Check sheet for the modelled part. Datum: model origin and axes. Units: mm. Round coordinates to 2 decimals unless told otherwise and drop trailing zeros. Write each loop counter-clockwise with the first axis right and the second up, starting at its lowest first coordinate (ties: lowest second). Pieces come first, ordered by that corner, then holes. Notation, with made-up numbers: M 85,11 L 127,11 A25 cw 127,33 Z; hole C -18.5,32.25 d2. An arc over 180 degrees is marked long. One line per item, written item: value.
Autodesk Inventor part; units mm, degrees
ref_plane "YZ Plane" through (0, 0, 0) normal (1, 0, 0) x (0, 1, 0)
ref_plane "XZ Plane" through (0, 0, 0) normal (0, 1, 0) x (-1, 0, 0)
ref_plane "XY Plane" through (0, 0, 0) normal (0, 0, 1) x (1, 0, 0)
sketch "Sketch1" plane through (0, 0, 0) normal (0, 0, 1) x (1, 0, 0)
  circle A0 centre (0, 5) radius 7.5
  line L0 (42.7333, 18.5) -> (-42.7333, 18.5)
  line L1 (-42.7333, -29) -> (42.7333, -29)
  circle A1 centre (18.5, 5) radius 2.25
  circle A2 centre (-18.5, 5) radius 2.25
  circle A3 centre (30.8333, 5) radius 3.9
  circle A4 centre (-30.8333, 5) radius 3.9
  line L2 (42.7333, 18.5) -> (42.7333, -29)
  line L3 (-42.7333, -29) -> (-42.7333, 18.5)
  circle A5 centre (0, 5) radius 13.5 construction
  line L4 (0, 41.7106) -> (0, -39.2634) construction
  dimension "d2" = 4.5
  dimension "d3" = 4.5
  dimension "d4" = 7.8
  dimension "d5" = 7.8
  dimension "d48" = 47.5
  dimension "d58" = 15
  dimension "d63" = 27
  dimension "d75" = 34
  dimension "d76" = 30.8333
  dimension "d77" = 85.4667
  dimension "d93" = 47.5
  dimension "d99" = 61.667
extrude "Extrusion1" add sketch "Sketch1" against normal blind 3
sketch "Sketch4" plane through (0, 0, 0) normal (0, 0, 1) x (1, 0, 0)
  line L0 (42.7333, 18.5) -> (39.7333, 18.5)
  line L1 (-42.7333, 18.5) -> (-39.7333, 18.5)
  line L2 (42.7333, -29) -> (21.3667, -29)
  line L3 (21.3667, -26) -> (39.7333, -26)
  line L4 (-42.7333, -29) -> (-21.3667, -29)
  line L5 (-21.3667, -29) -> (-21.3667, -26)
  line L6 (-21.3667, -26) -> (-39.7333, -26)
  line L7 (-42.7333, -23) -> (-42.7333, -29)
  line L8 (42.7333, 18.5) -> (39.7333, 18.5)
  line L9 (39.7333, 18.5) -> (39.7333, 2.6667)
  line L10 (39.7333, 2.6667) -> (42.7333, 2.6667)
  line L11 (42.7333, 2.6667) -> (42.7333, 18.5)
  line L12 (39.7333, -26) -> (39.7333, -13.1667)
  line L13 (39.7333, -13.1667) -> (42.7333, -13.1667)
  line L14 (-42.7333, 2.6667) -> (-39.7333, 2.6667)
  line L15 (-39.7333, 2.6667) -> (-39.7333, 18.5)
  line L16 (-39.7333, 18.5) -> (-42.7333, 18.5)
  line L17 (-42.7333, 18.5) -> (-42.7333, 2.6667)
  line L18 (-42.7333, -29) -> (-39.7333, -29)
  line L19 (-39.7333, -26) -> (-39.7333, -13.1667)
  line L20 (-39.7333, -13.1667) -> (-42.7333, -13.1667)
  line L21 (-42.7333, -13.1667) -> (-42.7333, -29)
  line L22 (21.3667, -29) -> (21.3667, -26)
  line L23 (-21.3667, -23) -> (-21.3667, -29)
  line L24 (-42.7333, 18.5) -> (-39.7333, 18.5)
  line L25 (-42.7333, -29) -> (42.7333, -29)
  line L26 (42.7333, 18.5) -> (-42.7333, 18.5)
  line L27 (50.1623, -5.25) -> (-50.4474, -5.25) construction
  line L28 (42.7333, -29) -> (42.7333, 18.5)
  line L29 (42.7333, -3.75) -> (34.7333, -3.75)
  line L30 (34.7333, -3.75) -> (34.7333, -6.75)
  line L31 (34.7333, -6.75) -> (42.7333, -6.75)
  line L32 (42.7333, -6.75) -> (42.7333, -3.75)
  circle A0 centre (0, 5) radius 13.5 construction
  circle A1 centre (0, 5) radius 7.5
  line L33 (42.7333, -2.6) -> (39.7333, -2.6)
  line L34 (39.7333, -2.6) -> (39.7333, -7.9)
  line L35 (39.7333, -7.9) -> (42.7333, -7.9)
  line L36 (42.7333, -7.9) -> (42.7333, -2.6)
  line L37 (35.3333, -2.6) -> (37.7333, -2.6)
  line L38 (37.7333, -2.6) -> (37.7333, -7.9)
  line L39 (37.7333, -7.9) -> (35.3333, -7.9)
  line L40 (35.3333, -7.9) -> (35.3333, -2.6)
  line L41 (0, 33.7344) -> (0, -36.9537) construction
  line L42 (-42.7333, 18.5) -> (-42.7333, -29)
  line L43 (-42.7333, -3.75) -> (-34.7333, -3.75)
  line L44 (-34.7333, -3.75) -> (-34.7333, -6.75)
  line L45 (-34.7333, -6.75) -> (-42.7333, -6.75)
  line L46 (-42.7333, -6.75) -> (-42.7333, -3.75)
  line L47 (-42.7333, -2.6) -> (-39.7333, -2.6)
  line L48 (-39.7333, -2.6) -> (-39.7333, -7.9)
  line L49 (-39.7333, -7.9) -> (-42.7333, -7.9)
  line L50 (-42.7333, -7.9) -> (-42.7333, -2.6)
  line L51 (-35.3333, -2.6) -> (-37.7333, -2.6)
  line L52 (-37.7333, -2.6) -> (-37.7333, -7.9)
  line L53 (-37.7333, -7.9) -> (-35.3333, -7.9)
  line L54 (-35.3333, -7.9) -> (-35.3333, -2.6)
  line L55 (42.7333, -29) -> (-42.7333, -29)
  line L56 (-1.5, -29) -> (1.5, -29)
  line L57 (1.5, -29) -> (1.5, -21)
  line L58 (1.5, -21) -> (-1.5, -21)
  line L59 (-1.5, -21) -> (-1.5, -29)
  line L60 (-2.65, -29) -> (2.65, -29)
  line L61 (2.65, -29) -> (2.65, -26)
  line L62 (2.65, -26) -> (-2.65, -26)
  line L63 (-2.65, -26) -> (-2.65, -29)
  line L64 (-2.65, -21.6) -> (2.65, -21.6)
  line L65 (2.65, -21.6) -> (2.65, -24)
  line L66 (2.65, -24) -> (-2.65, -24)
  line L67 (-2.65, -24) -> (-2.65, -21.6)
  line L68 (31.3, 16) -> (24.0167, 16) construction
  line L69 (11.4333, 16) -> (11.4333, 13) construction
  line L70 (11.4333, 13) -> (18.7167, 13) construction
  line L71 (31.3, 13) -> (31.3, 16) construction
  circle A2 centre (30.8333, 5) radius 3.9
  line L72 (21.3667, 17.602) -> (21.3667, 7.8585) construction
  line L73 (18.7167, 16) -> (24.0167, 16) construction
  line L74 (24.0167, 16) -> (24.0167, 13) construction
  line L75 (24.0167, 13) -> (18.7167, 13) construction
  line L76 (18.7167, 13) -> (18.7167, 16) construction
  line L77 (18.7167, 16) -> (11.4333, 16) construction
  line L78 (24.0167, 13) -> (31.3, 13) construction
  circle A3 centre (21.3667, 14.5) radius 1.4
  line L79 (-31.3, 16) -> (-24.0167, 16) construction
  line L80 (-11.4333, 16) -> (-11.4333, 13) construction
  line L81 (-11.4333, 13) -> (-18.7167, 13) construction
  line L82 (-31.3, 13) -> (-31.3, 16) construction
  line L83 (-24.0167, 16) -> (-24.0167, 13) construction
  line L84 (-18.7167, 13) -> (-18.7167, 16) construction
  line L85 (-18.7167, 16) -> (-11.4333, 16) construction
  line L86 (-24.0167, 13) -> (-31.3, 13) construction
  circle A4 centre (-21.3667, 14.5) radius 1.4
  line L87 (42.7333, 18.5) -> (42.7333, -29)
  line L88 (42.7333, -13.1667) -> (42.7333, -29)
  line L89 (11.4247, 13) -> (11.4247, 16)
  line L90 (11.4247, 16) -> (18.7077, 16)
  line L91 (18.7077, 16) -> (18.7077, 13)
  line L92 (18.7077, 13) -> (11.4247, 13)
  line L93 (31.2907, 16) -> (31.2907, 13)
  line L94 (31.2907, 13) -> (24.0077, 13)
  line L95 (24.0077, 13) -> (24.0077, 16)
  line L96 (24.0077, 16) -> (31.2907, 16)
  line L97 (-18.7073, 13) -> (-18.7073, 16)
  line L98 (-18.7073, 16) -> (-11.4243, 16)
  line L99 (-11.4243, 16) -> (-11.4243, 13)
  line L100 (-11.4243, 13) -> (-18.7073, 13)
  line L101 (-24.0073, 16) -> (-24.0073, 13)
  line L102 (-24.0073, 13) -> (-31.2903, 13)
  line L103 (-31.2903, 13) -> (-31.2903, 16)
  line L104 (-31.2903, 16) -> (-24.0073, 16)
  dimension "d25" = 3
  dimension "d26" = 3
  dimension "d33" = 15.8333
  dimension "d59" = 8
  dimension "d60" = 3
  dimension "d61" = 47.5
  dimension "d62" = 27
  dimension "d65" = 5.3
  dimension "d66" = 2.4
  dimension "d68" = 5
  dimension "d69" = 3
  dimension "d70" = 8
  dimension "d71" = 5.3
  dimension "d74" = 5
  dimension "d78" = 3
  dimension "d81" = 3
  dimension "d82" = 11
  dimension "d83" = 19.8667
  dimension "d85" = 79.4667
  dimension "d86" = 85.4667
  dimension "d87" = 3
  dimension "d88" = 5.3
  dimension "d89" = 2.8
  dimension "d91" = 15.8333
  dimension "d92" = 21.3667
  dimension "d94" = 2.4
  dimension "d95" = 2.4
  dimension "d96" = 11.4333
  dimension "d97" = 7.2833
  dimension "d98" = 2.65
extrude "Extrusion2" cut sketch "Sketch4" against normal through all contours L11 L10 L9 L0 | L15 L14 L17 L1 | L28 L29 L34 L33 | L28 L31 L34 L29 | L28 L35 L34 L31 | L34 L31 L38 L29 | L47 L48 L43 L42 | L38 L31 L40 L29 | L29 L40 L37 L38 | L43 L48 L45 L42 | L28 L2 L22 L3 L12 L13 | L38 L39 L40 L31 | L40 L31 L30 L29 | L45 L48 L49 L42 | L43 L52 L45 L48 | L52 L51 L54 L43 | L43 L54 L45 L52 | L20 L19 L6 L5 L4 L7 L21 | L45 L54 L53 L52 | L43 L44 L45 L54 | L25 L57 L62 L61 | L25 L59 L62 L57 | L25 L63 L62 L59 | L62 L59 L66 L57 | L66 L59 L64 L57 | L57 L64 L65 L66 | L66 L67 L64 L59 | L64 L59 L58 L57 | A1 | A3 | A4 | L89 L90 L91 L92 | L93 L94 L95 L96 | L97 L98 L99 L100 | L101 L102 L103 L104
equation "\"d48\" = d75 + 0.5 * d63"
equation "\"d33\" = 0.333333 * d61"
properties part number "X-Anchor_Front-Outer"
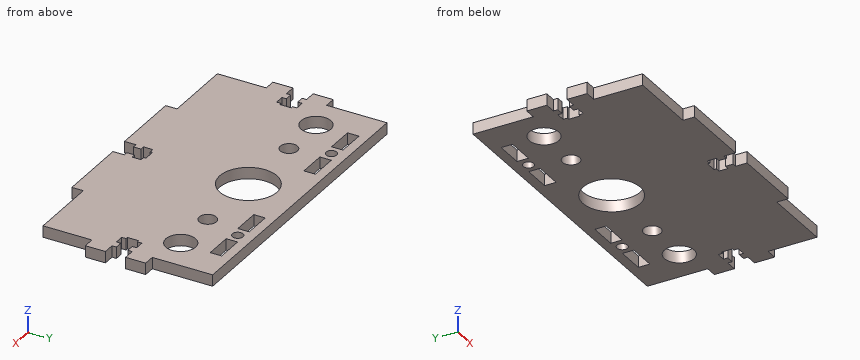
Q1. Sectioned sample at D-D on z = -0.55. State how many separate pieces and enclosed holes the cut face has, and give its area (3 significant figures).
Completed:
separate pieces: 1
enclosed holes: 11
area: 3,250 mm^2
Q2. Scan lines: line 1 (X direction, y = -3, z = -0.7); line 2 (Y direction, x = 18.5, z = -1.9); line 3 (X direction, y = 6, z = -2.6). Record each from-to range of solid material in increasing order. Write a range as [from, to].
Completed:
line 1: [-39.73, -37.73], [-35.33, 35.33], [37.73, 39.73]
line 2: [-29, 2.75], [7.25, 13], [16, 18.5]
line 3: [-39.73, -34.6], [-27.06, -20.52], [-16.48, -7.43], [7.43, 16.48], [20.52, 27.06], [34.6, 39.73]
Q3. Sectioned sample at B-B on x = -25.5. Enter the section's corners in (y, z).
Completed:
outline: M -26,-3 L 13,-3 L 13,0 L -26,0 Z; M 16,-3 L 18.5,-3 L 18.5,0 L 16,0 Z
Q4. Sectioned sample at A-A on x = 0. Enter the section's corners in (y, z).
Completed:
outline: M -21,-3 L -2.5,-3 L -2.5,0 L -21,0 Z; M 12.5,-3 L 18.5,-3 L 18.5,0 L 12.5,0 Z
Q5. Depth check by flat-ended pin: P1, Ø0.9, axis at y = -28, z = -1.5, coming from the -X side; P2, Ø0.9, axis at x = 2, z = -2, coming from the -Y side; P3, Ø0.9, axis at y = 15, z = -2, coming from the +X side. Enter the tip coordinate at first touch or a pass-through.
Completed:
P1: x = -21.37
P2: y = -26
P3: x = 39.73
Q6. Sectioned sample at C-C on y = -15. Enter the section's corners in (x, z).
Completed:
outline: M -39.73,-3 L 39.73,-3 L 39.73,0 L -39.73,0 Z
